Read the model definition and answer for the solid it produces. Units are mm, in the model's axes. Coordinates: 2 decimals unless noted, no trailing zeros. Loops run counter-clockwise (first coordinate to the right, second up) from the corner with the lowest first, then second, coordinate; pieces in that order, holes last. Notation, with made-up numbers: (42, -11) - (47, -11) arc R17 ccw to (47, 7) - close; hole circle Ø8 at (-33.5, 25.5). An arc over 180 degrees is marked (long way). Use CSV: the item, a comma, the result in double quotes.
Autodesk Inventor part; units mm, degrees
ref_plane "YZ Plane" through (0, 0, 0) normal (1, 0, 0) x (0, 1, 0)
ref_plane "XZ Plane" through (0, 0, 0) normal (0, 1, 0) x (-1, 0, 0)
ref_plane "XY Plane" through (0, 0, 0) normal (0, 0, 1) x (1, 0, 0)
sketch "Sketch1" plane through (0, 0, 0) normal (0, 1, 0) x (-1, 0, 0)
  line L0 (0, -7.3406) -> (-6.3571, -3.6703)
  line L1 (-6.3571, -3.6703) -> (-6.3571, 3.6703)
  line L2 (-6.3571, 3.6703) -> (0, 7.3406)
  line L3 (0, 7.3406) -> (6.3571, 3.6703)
  line L4 (6.3571, 3.6703) -> (6.3571, -3.6703)
  line L5 (6.3571, -3.6703) -> (0, -7.3406)
  point P0 (0, 0)
  point P1 (0, 0)
  dimension "d0" = 7.3406
extrude "Extrusion1" add sketch "Sketch1" along normal blind 93.98
properties part number "drive hex shaft"
Q1. The part is cut by section B-B on x = -2.75. Determine the outline of the cut face in (y, z).
Reported:
outline,"(0, -5.75) - (93.98, -5.75) - (93.98, 5.75) - (0, 5.75) - close"
Q2. The part is cut by section C-C on z = 4.5. Determine the outline of the cut face in (x, y), and give its area (3 significant figures).
Reported:
outline,"(-4.92, 0) - (4.92, 0) - (4.92, 93.98) - (-4.92, 93.98) - close"
area,"925 mm²"
Q3. Find the intervals of material crossed by probe 1 along X at (y, z) = (47, 6.5); probe 2 along Z at (x, y) = (2.75, 18); probe 3 along X at (y, z) = (58, -5.75), in increasing order. Write a range as [from, to].
Reported:
probe 1,"x = [-1.46, 1.46]"
probe 2,"z = [-5.75, 5.75]"
probe 3,"x = [-2.75, 2.75]"
Q4. Given P1, Ø6, axis at x = 0, z = -1, coming from the -Y side; P2, Ø5, axis at x = -3.5, y = 29.5, coming from the -Z side, each flat-ended and moving along its own axis, determine where each tip first touches the part or whether it passes through.
Reported:
P1,"stops at y = 0"
P2,"stops at z = -6.76"
Q5. The part is cut by section A-A on y = 74.5. Determine the outline of the cut face in (x, z), and give its area (3 significant figures).
Reported:
outline,"(-6.36, -3.67) - (0, -7.34) - (6.36, -3.67) - (6.36, 3.67) - (0, 7.34) - (-6.36, 3.67) - close"
area,"140 mm²"
